```python
from build123d import *

# Parameters (mm, degrees)
F4_W      = 39
F4_H      = 114
F5_DEPTH  = 43
F6_T      = -2
F7_W      = 35
F7_H      = 2
F8_DEPTH  = 6
F9_W      = 2.75
F9_H      = 2
F10_DEPTH = 2
F11_R     = 2
F13_DEPTH = 114.001
F14_R     = 3


with BuildPart() as f5:
    # F4 (on Top) → F5 (new body)
    with BuildSketch(Plane.XY):
        Rectangle(F4_W, F4_H)
    extrude(amount=F5_DEPTH)

    # F6
    f6_openings = [f5.faces().sort_by_distance(p)[0] for p in [
        (0, 0, 43),
    ]]
    offset(amount=F6_T, openings=f6_openings)

    # F7 (on face) → F8 (join)
    with BuildSketch(Plane.XY.offset(2)):
        with Locations((0, 36.5)):
            Rectangle(F7_W, F7_H)
        with Locations((0, -49)):
            Rectangle(F7_W, F7_H)
    extrude(amount=F8_DEPTH)

    # F9 (on face) → F10 (join)
    with BuildSketch(Plane.XY.offset(8)):
        with Locations((-16.125, 36.5)):
            Rectangle(F9_W, F9_H)
        with Locations((16.125, 36.5)):
            Rectangle(F9_W, F9_H)
        with Locations((-16.125, -49)):
            Rectangle(F9_W, F9_H)
        with Locations((16.125, -49)):
            Rectangle(F9_W, F9_H)
    extrude(amount=F10_DEPTH)

    # F11
    f11_edges = [f5.edges().sort_by_distance(p)[0] for p in [
        (-17.5, 55, 22.5),
        (-17.5, 46.25, 2),
        (0, 55, 2),
        (-17.5, -6.25, 2),
        (0, -48, 2),
        (-17.5, -52.5, 2),
        (0, -50, 2),
        (0, -55, 2),
        (-17.5, -55, 22.5),
        (17.5, -55, 22.5),
        (17.5, -52.5, 2),
        (17.5, -6.25, 2),
        (0, 37.5, 2),
        (0, 35.5, 2),
        (17.5, 46.25, 2),
        (17.5, 55, 22.5),
    ]]
    fillet(f11_edges, radius=F11_R)

    # F12 (on face) → F13 (cut, through all)
    with BuildSketch(Plane.XZ.offset(57)):
        with BuildLine():
            Line((-5, 43), (-5, 38))
            ThreePointArc((-5, 38), (-3.5355339142, 41.5355338977), (-2.33e-08, 43))
            Line((-2.33e-08, 43), (-5, 43))
        make_face()
        with BuildLine():
            ThreePointArc((-5, 38), (-3.5355339059, 34.4644660941), (0, 33))
            ThreePointArc((0, 33), (3.5355339059, 34.4644660941), (5, 38))
            ThreePointArc((5, 38), (3.5355338977, 41.5355339142), (-2.33e-08, 43))
            ThreePointArc((-2.33e-08, 43), (-3.5355339142, 41.5355338977), (-5, 38))
        make_face()
        with BuildLine():
            ThreePointArc((-2.33e-08, 43), (3.5355338977, 41.5355339142), (5, 38))
            Line((5, 38), (5, 43))
            Line((5, 43), (-2.33e-08, 43))
        make_face()
    extrude(amount=-F13_DEPTH, mode=Mode.SUBTRACT)

    # F14
    f14_edges = [f5.edges().sort_by_distance(p)[0] for p in [
        (19.5, -57, 21.5),
        (19.5, 57, 21.5),
        (-19.5, 57, 21.5),
        (-19.5, -57, 21.5),
    ]]
    fillet(f14_edges, radius=F14_R)


solid = f5.part
```
Can you work these out from the model? Positions are in its coordinate system, mm. A direction names the side the tool comes from. Coordinates: 2 decimals unless noted, no trailing zeros. Write each loop counter-clockwise with the first axis right and the second up, starting at its lowest first coordinate (ties: lowest second). Pieces come first, ordered by that corner, then holes. Notation, with made-up numbers: M -34,59.25 L 12,59.25 A27 cw 12,78.25 Z; hole C 55,50.5 d2. An arc over 180 degrees is marked long. Write item = value, one per line. Start each with the question number.
Q1. On a 3-axis mill with a long thin cutter (end or side, diameter ignored), from which of +Z, -Z, +X, -X, +Y, -Y can I reach the whole of each face in a straight line? I mean faces 1 (the face through (19.5, -1, 21)), 2 (the face through (0, -49, 8)). Say none if no direction works.
Q2. Thinking about a two-plate mould opening in Y: for faces 3 (the face through (16.9, -5.67, 2.57)), 4 (the face through (0, 55, 23)), 5 (the face through (-18.64, 56.1, 21.8)), 6 (the face through (5, -56, 40)), which applies, released by +Y, released by -Y, zero draft, split by the parting line, or undercut?
Q3. If we section it at B-B, the plane y = -5.5: Write out the boundary of the cut face in (x, z), then the cut area to 3 significant figures.
Q4. If I drill on L1, parallel to Y at x = -10, z = 6; L2, parallel to Y at x = 11, z = 34; L3, parallel to X at y = 47, z = 40, over which ranges is the centre line in solid material (lowest first)? Write a range as [from, to].
Q5. If we section it at A-A, the plane z = 16: Write out the boundary of the cut face in (x, y), then the cut area to 3 significant figures.
Q6. If we section it at C-C, the plane x = 13.5: Write out the boundary of the cut face in (y, z).
Q7. I'm going to push flat-ended pins straight in: pin 1 (7 mm diameter, centred on x = 1.5, y = 48, fed in from +Z); pin 2 (2 mm diameter, centred on x = -4.5, y = 37, fed in from +Z); pin 3 (2 mm diameter, centred on y = -56.5, z = 40, fed in from -X). Where does each tip first touch, or does it pass through?
Check sheet entries:
q1.face_1 = +Z, -Z, +X, +Y, -Y
q1.face_2 = +Z
q2.face_3 = undercut
q2.face_4 = undercut
q2.face_5 = released by +Y
q2.face_6 = zero draft
q3.outline = M -19.5,0 L 19.5,0 L 19.5,43 L 17.5,43 L 17.5,4 A2 cw 15.5,2 L -15.5,2 A2 cw -17.5,4 L -17.5,43 L -19.5,43 Z
q3.area = 244 mm²
q4.L1 = [-57, -55], [-50, -48], [35.5, 37.5], [55, 57]
q4.L2 = [-57, -55], [55, 57]
q4.L3 = [-19.5, -17.5], [17.5, 19.5]
q5.outline = M -19.5,-54 A3 ccw -16.5,-57 L 16.5,-57 A3 ccw 19.5,-54 L 19.5,54 A3 ccw 16.5,57 L -16.5,57 A3 ccw -19.5,54 Z; hole M -17.5,-53 A2 ccw -15.5,-55 L 15.5,-55 A2 ccw 17.5,-53 L 17.5,53 A2 ccw 15.5,55 L -15.5,55 A2 ccw -17.5,53 Z
q5.area = 592 mm²
q6.outline = M -57,0 L 57,0 L 57,43 L 55,43 L 55,4 A2 cw 53,2 L 39.5,2 A2 cw 37.5,4 L 37.5,8 L 35.5,8 L 35.5,4 A2 cw 33.5,2 L -46,2 A2 cw -48,4 L -48,8 L -50,8 L -50,4 A2 cw -52,2 L -53,2 A2 cw -55,4 L -55,43 L -57,43 Z
q7.pin_1 = 2
q7.pin_2 = 8
q7.pin_3 = -19.1
